Geometry: final body of the model. Coordinates: model frame, mm. Face numbers are marked on the shaded views. A direction names the side the tool comes from. Give positions to 0.01 mm unless a question says otherwise; leave off trailing zeros. Loops run counter-clockwise (first coordinate to the right, second up) from the corner with the lowest first, then second, coordinate; pieces in that order, holes last.
1. Access query for the marked faces 1, 2 and 3. Directions: +Z, -Z, +X, -X, +Y, -Y. A direction counts if a zero-diameter tool reaches every point of the face in a straight line with its end or side. Return the directions, or none.
2. Material intervals for line 1 along Z through (x, y) = (2, 3.25); line 2 along Y through (x, z) = (16.1, -70.5); line 3 along Y through (x, z) = (21, -35.5), sorted ascending.
3. Section B-B, the plane y = 15. Output: boundary loops of the cut face in (x, z).
4. First-contact query: P1, Ø2.5, axis at x = -1, y = 2, coming from the +Z side; P2, Ø5, axis at y = 2.5, z = -17, coming from the -X side; P3, Ø1, axis at y = 10.5, z = -5.5, coming from the -X side; P4, Ø4, axis at y = 11.5, z = -70.5, coming from the -X side. Flat tips, straight axial feed; report the tip coordinate or a pass-through.
5. Section C-C, the plane z = -54. Output: boundary loops of the cut face in (x, y), then the cut area to 3 significant figures.
6. Section D-D, the plane x = 9.5. Output: boundary loops of the cut face in (y, z), then the cut area to 3 significant figures.
7. Draft query along X for the marked faces 4, 5, 6 and 7. Return one class per face: +X half, -X half, draft (parallel to the pull), parting line (faces both ways), or undercut.
8. Section A-A, the plane z = 4.5. Output: boundary loops of the cut face in (x, y), then the cut area to 3 significant figures.
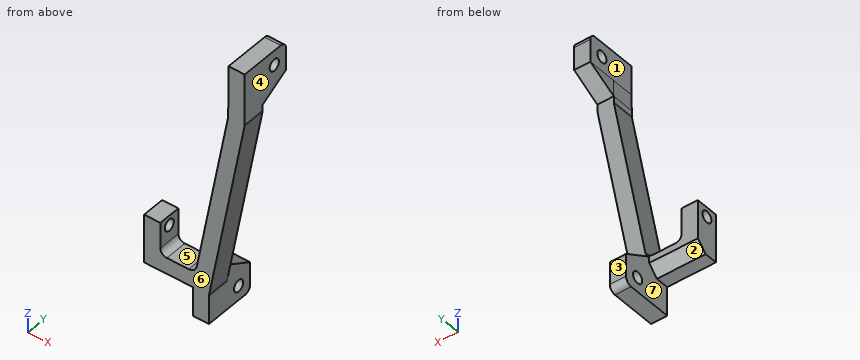
from build123d import *

# Parameters (mm, degrees)
BOSS_EXTRUDE1_DEPTH  = 7
BOSS_EXTRUDE2_START  = 7
SKETCH1_3_W          = 5
SKETCH1_3_H          = 9
BOSS_EXTRUDE2_DEPTH  = 9
M3_CLEARANCE_HOLE1_D = 3.6
FILLET2_R            = 2.5
CHAMFER3_SIZE        = 5
CHAMFER3_SIZE_2      = 9.020238776
CHAMFER2_SIZE        = 3
SKETCH6_W            = 5
SKETCH6_H            = 7
BOSS_EXTRUDE3_DEPTH  = 10
SKETCH7_R            = 1.75
CUT_EXTRUDE1_DEPTH   = 10
FILLET6_R            = 2
SKETCH8_W            = 84
SKETCH8_H            = 16
CUT_EXTRUDE2_DEPTH   = 26
FILLET8_R            = 2


with BuildPart() as part:
    # Sketch1 → Boss-Extrude1 (new body)
    with BuildSketch(Plane(origin=(0, 0, 0), x_dir=(1, 0, 0), z_dir=(0, 1, 0))):
        Polygon((-23.5, -9), (-23.5, 0), (-23.413842004, 5), (-23.413842004, 7), (-13.346045394, 61), (13.346045394, 61), (23.413842004, 7), (23.413842004, 5), (23.5, 0), (23.5, -9), (28.5, -9), (28.5, 7), (17.5, 66), (17.5, 75), (12.5, 75), (12.5, 66), (-12.5, 66), (-12.5, 75), (-17.5, 75), (-17.5, 66), (-28.5, 7), (-28.5, -9), align=None)
    extrude(amount=BOSS_EXTRUDE1_DEPTH)

    # Sketch1<3> → Boss-Extrude2 (add)
    with BuildSketch(Plane(origin=(0, 0, 0), x_dir=(1, 0, 0), z_dir=(0, 1, 0)).offset(BOSS_EXTRUDE2_START)):
        with Locations((-15, 70.5)):
            Rectangle(SKETCH1_3_W, SKETCH1_3_H)
        with Locations((15, 70.5)):
            Rectangle(SKETCH1_3_W, SKETCH1_3_H)
        with Locations((-26, -4.5)):
            Rectangle(SKETCH1_3_W, SKETCH1_3_H)
        with Locations((26, -4.5)):
            Rectangle(SKETCH1_3_W, SKETCH1_3_H)
    extrude(amount=BOSS_EXTRUDE2_DEPTH)

    # M3 Clearance Hole1 (through all)
    with Locations(Plane(origin=(28.5, 0, 0), x_dir=(0, 0, -1), z_dir=(1, 0, 0))):
        with Locations((-4.5, 11.5), (70.5, 11.5)):
            Hole(M3_CLEARANCE_HOLE1_D / 2)

    # Fillet2
    fillet2_edges = [part.edges().sort_by_distance(p)[0] for p in [
        (-28.5, 3.5, -7),
        (-17.5, 3.5, -66),
        (17.5, 3.5, -66),
        (28.5, 3.5, -7),
        (23.413842004, 3.5, -5),
        (23.413842004, 3.5, -7),
        (13.346045394, 3.5, -61),
        (-13.346045394, 3.5, -61),
        (-23.413842004, 3.5, -7),
        (-23.413842004, 3.5, -5),
    ]]
    fillet(fillet2_edges, radius=FILLET2_R)

    # Chamfer3
    # the kernel refuses this chamfer: 9.020238776, 5 mm, written as the material it adds along each edge
    with BuildSketch(Plane(origin=(0.156378648, 7, 0), x_dir=(1.7315070193455174e-15, -0.060867759165289366, -0.9981458389905739), z_dir=(1, 0, 0))) as chamfer3_piece_1_section:
        Polygon((CHAMFER3_SIZE * 0.998145838991, CHAMFER3_SIZE * 0.0608677591653), (-CHAMFER3_SIZE_2 * 0.0608677591677, CHAMFER3_SIZE_2 * 0.99814583903), (0, 0), align=None)
    chamfer3_piece_1 = extrude(amount=28.343621352, mode=Mode.PRIVATE)
    chamfer3_piece_1 = split(chamfer3_piece_1, bisect_by=Plane(origin=(23.456927395, 9.255059618, -2.499628978), z_dir=(0.9998515690487569, 0, -0.017229041492165368)), keep=Keep.TOP, mode=Mode.PRIVATE)
    chamfer3_piece_1 = split(chamfer3_piece_1, bisect_by=Plane(origin=(23.478460501, 16, -2.500000028), z_dir=(0, -1, 0)), keep=Keep.TOP, mode=Mode.PRIVATE)
    add(chamfer3_piece_1)
    with BuildSketch(Plane(origin=(12.5, 7, -66), x_dir=(0, -0.06086775916528939, 0.9981458389905739), z_dir=(1, 0, 0))) as chamfer3_piece_2_section:
        Polygon((CHAMFER3_SIZE * 0.998145838991, -CHAMFER3_SIZE * 0.0608677591653), (-CHAMFER3_SIZE_2 * 0.0608677591677, -CHAMFER3_SIZE_2 * 0.99814583903), (0, 0), align=None)
    chamfer3_piece_2 = extrude(amount=5, mode=Mode.PRIVATE)
    chamfer3_piece_2 = split(chamfer3_piece_2, bisect_by=Plane(origin=(15, 16, -64.333324962), z_dir=(0, -1, 0)), keep=Keep.TOP, mode=Mode.PRIVATE)
    add(chamfer3_piece_2)

    # Chamfer2
    chamfer2_edges = [part.edges().sort_by_distance(p)[0] for p in [
        (0, 7, -66),
    ]]
    chamfer(chamfer2_edges, length=CHAMFER2_SIZE)

    # Sketch6 → Boss-Extrude3 (add)
    with BuildSketch(Plane(origin=(0, 0, -61), x_dir=(-1, 0, 0), z_dir=(0, 0, 1))):
        with Locations((0, -3.5)):
            Rectangle(SKETCH6_W, SKETCH6_H)
    extrude(amount=BOSS_EXTRUDE3_DEPTH)

    # Sketch7 → Cut-Extrude1 (cut)
    with BuildSketch(Plane(origin=(2.5, 0, 0), x_dir=(0, 0, -1), z_dir=(1, 0, 0))):
        with Locations((54, 3.5)):
            Circle(SKETCH7_R)
    extrude(amount=-CUT_EXTRUDE1_DEPTH, mode=Mode.SUBTRACT)

    # Fillet6
    fillet6_edges = [part.edges().sort_by_distance(p)[0] for p in [
        (26, 16, 9),
        (-15, 16, -75),
        (15, 16, -75),
        (-26, 16, 9),
    ]]
    fillet(fillet6_edges, radius=FILLET6_R)

    # Sketch8 → Cut-Extrude2 (cut)
    with BuildSketch(Plane.ZY.offset(28.5)):
        with Locations((-33, 8)):
            Rectangle(SKETCH8_W, SKETCH8_H)
    extrude(amount=-CUT_EXTRUDE2_DEPTH, mode=Mode.SUBTRACT)

    # Fillet8
    fillet8_edges = [part.edges().sort_by_distance(p)[0] for p in [
        (2.5, 3.5, -61),
    ]]
    fillet(fillet8_edges, radius=FILLET8_R)


solid = part.part
Answers below:
1. face 1: +Z, -X, +Y, -Y
1. face 2: -Z, -X, +Y
1. face 3: +Z, -Z, +X, -X, +Y
2. line 1: z = -66 to -55.73, -52.27 to -51
2. line 2: y = 0 to 9.7, 13.3 to 16
2. line 3: y = 0 to 7
3. outline: (12.5, -74.73) - (17.5, -74.73) - (17.5, -65.43) - (12.5, -65.43) - close; (23.49, -0.57) - (28.5, -0.57) - (28.5, 8.73) - (23.5, 8.73) - (23.5, 0) - close
4. P1: stops at z = -51
4. P2: stops at x = 21.08
4. P3: passes through
4. P4: stops at x = 12.5
5. outline: (-2.5, 0) - (2.5, 0) - (2.5, 1.75) - (-2.5, 1.75) - close; (-2.5, 5.25) - (2.5, 5.25) - (2.5, 7) - (-2.5, 7) - close; (14.65, 0) - (19.74, 0) - (19.74, 7) - (14.65, 7) - close
5. area: 53.1 mm2
6. outline: (0, -66) - (4, -66) - (7, -63) - (7, -61) - (0, -61) - close
6. area: 30.5 mm2
7. face 4: +X half
7. face 5: undercut
7. face 6: draft
7. face 7: -X half
8. outline: (23.5, 0) - (28.5, 0) - (28.5, 9.7) - (23.5, 9.7) - close; (23.5, 13.3) - (28.5, 13.3) - (28.5, 16) - (23.5, 16) - close
8. area: 62.0 mm2
